Input: part model. Units: mm. Frame: model coordinates. A direction names the side the tool comes from. Coordinates: 2 decimals unless noted, no trailing zeros. Order: outer loops, then holes, each group sorted by start corner. A loop starts at its lowest first (then second) coordinate and runs counter-clockwise, first axis right, second up. Notation, with made-up numbers: M 37,26 L 95,26 A22 ccw 95,65 Z; hole C -25,-2 d9. An arc over 180 degrees is marked long. One line per item, written item: value.
```python
from build123d import *

# Parameters (mm, degrees)
SKETCH1_W                  = 42
SKETCH1_H                  = 45
BOSS_EXTRUDE1_DEPTH        = 42
SKETCH2_R                  = 18
BOSS_EXTRUDE2_DEPTH        = 43.2
SKETCH3_R                  = 11
BOSS_EXTRUDE3_DEPTH        = 2
SKETCH4_R                  = 4
BOSS_EXTRUDE4_DEPTH        = 18
CUT_EXTRUDE1_START         = -15
CUT_EXTRUDE1_DEPTH         = 15
M2_CLEARANCE_HOLE1_D       = 2.459
M2_CLEARANCE_HOLE1_DEPTH   = 4
M3_5_CLEARANCE_HOLE1_D     = 4.134
M3_5_CLEARANCE_HOLE1_DEPTH = 5
CHAMFER1_SIZE              = 3
CHAMFER2_SIZE              = 0.5


with BuildPart() as part:
    # Sketch1 → Boss-Extrude1 (new body)
    with BuildSketch(Plane(origin=(0, 42, 0), x_dir=(1, 0, 0), z_dir=(0, 1, 0))):
        with Locations((21, -22.5)):
            Rectangle(SKETCH1_W, SKETCH1_H)
    extrude(amount=-BOSS_EXTRUDE1_DEPTH)

    # Sketch2 → Boss-Extrude2 (add)
    with BuildSketch(Plane.XY.offset(45)):
        with Locations(Location((20.992732048, 21.029062271, 0), (0, 0, 180))):
            Circle(SKETCH2_R)
    extrude(amount=BOSS_EXTRUDE2_DEPTH)

    # Sketch3 → Boss-Extrude3 (add)
    with BuildSketch(Plane.XY.offset(88.2)):
        with Locations((20.992732048, 21.029062271)):
            Circle(SKETCH3_R)
    extrude(amount=BOSS_EXTRUDE3_DEPTH)

    # Sketch4 → Boss-Extrude4 (add)
    with BuildSketch(Plane.XY.offset(90.2)):
        with Locations((20.992732048, 21.029062271)):
            Circle(SKETCH4_R)
    extrude(amount=BOSS_EXTRUDE4_DEPTH)

    # Sketch5 → Cut-Extrude1 (cut)
    with BuildSketch(Plane.XY.offset(108.2).offset(CUT_EXTRUDE1_START)):
        with BuildLine():
            Line((17.987520214, 18.389232384), (18.004545147, 23.688148401))
            ThreePointArc((18.004545147, 23.688148401), (16.992752693, 21.041913839), (17.987520214, 18.389232384))
        make_face()
    extrude(amount=CUT_EXTRUDE1_DEPTH, mode=Mode.SUBTRACT)

    # M2 Clearance Hole1
    with Locations(Plane.XY.offset(88.2)):
        with Locations((11.075764894, 30.962638855), (30.85750103, 30.962638855), (11.075764894, 11.143120527), (30.85750103, 11.143120527)):
            Hole(M2_CLEARANCE_HOLE1_D / 2, depth=M2_CLEARANCE_HOLE1_DEPTH)

    # M3.5 Clearance Hole1
    with Locations(Plane.XY.offset(88.2)):
        with Locations((6.992732048, 21.029062271), (34.992732048, 21.029062271), (20.992732048, 7.029062271), (20.992732048, 35.029062271)):
            Hole(M3_5_CLEARANCE_HOLE1_D / 2, depth=M3_5_CLEARANCE_HOLE1_DEPTH)

    # Chamfer1
    chamfer1_edges = [part.edges().sort_by_distance(p)[0] for p in [
        (0, 0, 22.5),
        (42, 0, 22.5),
        (0, 42, 22.5),
        (42, 42, 22.5),
    ]]
    chamfer(chamfer1_edges, length=CHAMFER1_SIZE)

    # Chamfer2
    chamfer2_edges = [part.edges().sort_by_distance(p)[0] for p in [
        (38.992732048, 21.029062271, 88.2),
        (22.403255473, 17.286012222, 108.2),
        (17.996032681, 21.038690392, 108.2),
    ]]
    chamfer(chamfer2_edges, length=CHAMFER2_SIZE)


solid = part.part
```
(1) Access query for faces 1 (the flat face through (31, 31, 84.2)), 2 (the flat face through (41, 2, 23)). Directions: +Z, -Z, +X, -X, +Y, -Y. A direction counts if a zero-diameter tool reaches every point of the face in a straight line with its end or side. Return the directions, or none.
Data:
face 1: +Z
face 2: +Z, -Z, +X, -Y
(2) Draft query along X for faces 3 (the flat face through (2, 41, 23)), 4 (the flat face through (11, 11, 84.2)), 5 (the cylindrical face through (19.561, 31.935, 89.186)). Return one class per face: released by +X, released by -X, zero draft, split by the parting line, or undercut.
Data:
face 3: released by -X
face 4: undercut
face 5: split by the parting line
(3) Cut plane A-A on z = 86. Give the number of separate pieces and of enclosed holes in the cut face, plus the area to 3 significant figures.
Data:
separate pieces: 1
enclosed holes: 8
area: 945 mm2
(4) Ray query, line 1 (Z direction, x = 8, y = 2.5); line 2 (Z direction, x = 4, y = 23.5); line 3 (X direction, y = 39.5, z = 40). Return the intervals inside material, ascending. Write a range as from..to.
Data:
line 1: z = 0..45
line 2: z = 0..88.2
line 3: x = 0.5..41.5
(5) Cut plane B-B on z = 68.5. Output: boundary loops of the cut face in (x, y).
Data:
outline: C 20.99,21.03 d36
(6) First-contact query: pin 1 (2 mm diameter, centred on x = 32, y = 10.5, fed in from +Z); pin 2 (0.5 mm diameter, centred on x = 17.5, y = 20, fed in from +Z); pin 3 (2 mm diameter, centred on x = 35.5, y = 21, fed in from +Z). Flat tips, straight axial feed; report the tip coordinate or a pass-through.
Data:
pin 1: stops at z = 88.2
pin 2: stops at z = 93.2
pin 3: stops at z = 83.2
